Work out the finished part from the listing and answer in its coordinate system (mm). A direction names the side the tool comes from. Round coordinates to 2 decimals unless told otherwise and drop trailing zeros. Order: outer loops, then holes, each group sorted by start corner. A loop starts at its lowest first (then second) coordinate and runs counter-clockwise, first axis right, second up. Notation, with made-up numbers: (75.25, 67) -> (121.25, 67) arc R26 ccw to (121.25, 81) -> close; hole circle Ø8 at (71.5, 60). An arc over 180 degrees is marked (long way). Use one line per item in the form item = value.
```python
from build123d import *

# Parameters (mm, degrees)
ESQUISSE1_R             = 30
BOSS_EXTRU_1_DEPTH      = 101
ESQUISSE2_R             = 4
BOSS_EXTRU_2_DEPTH      = 20
ENL_V_START             = -10
ENL_V_MAT_EXTRU_1_DEPTH = 10
CONG_1_R                = 1
ESQUISSE4_R             = 17
BOSS_EXTRU_3_DEPTH      = 9
ESQUISSE5_R             = 2.25
ENL_V_MAT_EXTRU_2_DEPTH = 9
ESQUISSE7_W             = 20
ESQUISSE7_H             = 79


with BuildPart() as part:
    # Esquisse1 → Boss.-Extru.1 (new body)
    with BuildSketch(Plane(origin=(0, 0, 0), x_dir=(0, 1, 0), z_dir=(0, 0, 1))):
        with Locations(Location((0, 0, 0), (0, 0, 270))):
            Circle(ESQUISSE1_R)
    extrude(amount=BOSS_EXTRU_1_DEPTH)

    # Esquisse2 → Boss.-Extru.2 (add)
    with BuildSketch(Plane.XY.offset(101)):
        Circle(ESQUISSE2_R)
    extrude(amount=BOSS_EXTRU_2_DEPTH)

    # Esquisse3 → Enlèv. mat.-Extru.1 (cut)
    with BuildSketch(Plane.XY.offset(121).offset(ENL_V_START)):
        with BuildLine():
            Line((-3.142677151, 2.4745869), (3.101981411, 2.5254131))
            ThreePointArc((3.101981411, 2.5254131), (-0.032555514, 3.999867515), (-3.142677151, 2.4745869))
        make_face()
    extrude(amount=ENL_V_MAT_EXTRU_1_DEPTH, mode=Mode.SUBTRACT)

    # Congé1
    cong_1_edges = [part.edges().sort_by_distance(p)[0] for p in [
        (-30, 0, 0),
        (-30, 0, 101),
    ]]
    fillet(cong_1_edges, radius=CONG_1_R)

    # Esquisse4 → Boss.-Extru.3 (add)
    with BuildSketch(Plane(origin=(0, 0, 0), x_dir=(1, 0, 0), z_dir=(0, 0, -1))):
        Circle(ESQUISSE4_R)
    extrude(amount=BOSS_EXTRU_3_DEPTH)

    # Esquisse5 → Enlèv. mat.-Extru.2 (cut)
    with BuildSketch(Plane.XY.offset(101)):
        with Locations((0, 22)):
            Circle(ESQUISSE5_R)
        with Locations((22, 0)):
            Circle(ESQUISSE5_R)
        with Locations((0, -22)):
            Circle(ESQUISSE5_R)
        with Locations((-22, 0)):
            Circle(ESQUISSE5_R)
    extrude(amount=-ENL_V_MAT_EXTRU_2_DEPTH, mode=Mode.SUBTRACT)

    # Esquisse7 → Enlèvement de matière-Révolution1 (revolve, cut)
    with BuildSketch(Plane.YZ, mode=Mode.PRIVATE) as enl_vement_de_mati_re_r_volution1_sk:
        with Locations((-10, 50.5)):
            Rectangle(ESQUISSE7_W, ESQUISSE7_H)
    revolve(enl_vement_de_mati_re_r_volution1_sk.sketch.rotate(Axis((0, 0, 90), (0, 0, -1)), 128.217378369), axis=Axis((0, 0, 90), (0, 0, -1)), mode=Mode.SUBTRACT)


solid = part.part
```
Item 1: Consider line 1 along X through (y, z) = (-0.5, 78); line 2 along Y through (x, z) = (0, 34.5); line 3 along Z through (x, y) = (5, 17.5). Determine where each line is inside the solid, lowest interval first.
Findings:
line_1 = -30 to -19.99, 19.99 to 30
line_2 = -30 to -20, 20 to 30
line_3 = 0 to 11, 90 to 101
Item 2: Flat-ended cylindrical pins translate along their axes: P1, Ø3.5, axis at x = -22, y = 0, coming from the -Z side; P2, Ø5, axis at x = 21.5, y = 1, coming from the +Z side; P3, Ø1.3, axis at x = -21.5, y = 0.5, coming from the +Z side. Find the tip coordinate at first contact, or state that the pin passes through.
Findings:
P1 = 0
P2 = 101
P3 = 92
Item 3: For faces 1 (the flat face through (0, 0, 11)), 2 (the flat face through (0, 0, -9)), 3 (the cylindrical face through (9.139, -14.334, -4.437)), 4 (the cylindrical face through (-0.867, -3.905, 110.86)), determine the directions among +Z, -Z, +X, -X, +Y, -Y from which every point of the face is accessible in a straight line to the end or side of a thin tool.
Findings:
face_1 = none
face_2 = -Z, +X, -X, +Y, -Y
face_3 = -Z
face_4 = +Z
Item 4: Determine the mould class of faces 5 (the cylindrical face through (-29.97, 1.32, 49.81)), 6 (the cylindrical face through (-11.3, 16.5, 51.1)), 7 (the flat face through (0, -1, 121)) for opening direction X: released by +X, released by -X, zero draft, split by the parting line, or undercut.
Findings:
face_5 = split by the parting line
face_6 = undercut
face_7 = zero draft
Item 5: The part is cut by section C-C, the plane z = 34. Give the vertices of the cut face in (x, y), and give its area (3 significant figures).
Findings:
outline = circle Ø60 at (0, 0); hole circle Ø40 at (0, 0)
area = 1,570 mm^2
Item 6: The part is cut by section A-A, the plane y = 0. Give the vertices of the cut face in (x, z).
Findings:
outline = (-30, 1) arc R1 ccw to (-29, 0) -> (-17, 0) -> (-17, -9) -> (17, -9) -> (17, 0) -> (29, 0) arc R1 ccw to (30, 1) -> (30, 100) arc R1 ccw to (29, 101) -> (24.25, 101) -> (24.25, 92) -> (19.75, 92) -> (19.75, 101) -> (4, 101) -> (4, 121) -> (-4, 121) -> (-4, 101) -> (-19.75, 101) -> (-19.75, 92) -> (-24.25, 92) -> (-24.25, 101) -> (-29, 101) arc R1 ccw to (-30, 100) -> close; hole (-20, 11) -> (20, 11) -> (20, 90) -> (-20, 90) -> close
